```python
from build123d import *

# Parameters (mm, degrees)
F1_DEPTH = 50
F3_D     = 10
F4_SIZE  = 5
F5_SIZE  = 5.08


with BuildPart() as f1:
    # F0 (on Front) → F1 (new body)
    with BuildSketch(Plane.XZ):
        Polygon((50, 68.819096), (-50, 68.819096), (-80.901699, -26.286556), (0, -85.065081), (80.901699, -26.286556), align=None)
    extrude(amount=F1_DEPTH)

    # F3 (through all)
    with Locations(Plane(origin=(0, 0, 0), x_dir=(-1, 0, 0), z_dir=(0, 1, 0))):
        with Locations((0, 0)):
            Hole(F3_D / 2)

    # F4
    f4_edges = [f1.edges().sort_by_distance(p)[0] for p in [
        (-50, -25, 68.819096),
    ]]
    chamfer(f4_edges, length=F4_SIZE)

    # F5
    f5_edges = [f1.edges().sort_by_distance(p)[0] for p in [
        (50, -25, 68.819096),
    ]]
    chamfer(f5_edges, length=F5_SIZE)


solid = f1.part
```
Can you work these out from the model? Positions are in its coordinate system, mm. Give positions to 0.01 mm unless a question says otherwise; leave off trailing zeros. Order: outer loops, then holes, each group sorted by start corner. A loop starts at its lowest first (then second) coordinate and runs counter-clockwise, first axis right, second up. Notation, with made-up numbers: M 77.5,29.25 L 96.5,29.25 A30 ccw 96.5,61.25 Z; hole C 26,3 d8. An arc over 180 degrees is marked long. Write item = value, one per line. Start each with the question number.
Q1. Will these pins go through, and if not, where does the flat tip stop? pin 1 Ø2 at (y, z) = (-21, 6) entering from -X; pin 2 Ø8 at (x, z) = (-43, 24) entering from +Y; pin 3 Ø6 at (x, y) = (11, -26.5) entering from -Z; pin 4 Ø4 at (y, z) = (-18.5, -64) entering from +X.
Q2. Suppose I cut it at B-B (y = -7.5). Write out the boundary of the cut face in (x, z).
Q3. We'd pull the mould along X, two halves only. Please class faces 1 (the flat face through (66.44, -24.65, 18.22)), 2 (the cylindrical face through (-1.08, -25.35, -4.88)), 3 (the flat face through (1, -25, 68.819)): pulls with the +X half, pulls with the -X half, needs draft (parallel to the pull), parting line crosses it, or undercut.
Q4. Suppose I cut it at C-C (x = 53.5). Write out the boundary of the cut face in (y, z).
Q5. Suppose I cut it at A-A (z = 0). Write out the boundary of the cut face in (x, y), plus the area to 3 significant figures.
Q6. Suppose I cut it at D-D (z = 29.5). Write out the boundary of the cut face in (x, y).
Q7. I need wall thicknesses on probe 1 along Z at (x, y) = (0, -10); probe 2 along Z at (x, y) = (4.5, -21); probe 3 along Z at (x, y) = (-24.5, -31.5). Which ranges of each line are inside material? Lowest first, please. Write a range as [from, to].
Check result:
q1.pin_1 = -70.74
q1.pin_2 = 0
q1.pin_3 = -79.25
q1.pin_4 = 31.75
q2.outline = M -80.9,-26.29 L 0,-85.07 L 80.9,-26.29 L 51.57,63.99 L 44.92,68.82 L -45,68.82 L -51.55,64.06 Z; hole C 0,0 d10
q3.face_1 = pulls with the +X half
q3.face_2 = undercut
q3.face_3 = needs draft
q4.outline = M -50,-46.2 L 0,-46.2 L 0,58.05 L -50,58.05 Z
q5.outline = M -72.36,-50 L -5,-50 L -5,0 L -72.36,0 Z; M 5,-50 L 72.36,-50 L 72.36,0 L 5,0 Z
q5.area = 6,740 mm2
q6.outline = M -62.78,-50 L 62.78,-50 L 62.78,0 L -62.78,0 Z
q7.probe_1 = [-85.07, -5], [5, 68.82]
q7.probe_2 = [-81.8, -2.18], [2.18, 68.82]
q7.probe_3 = [-67.26, 68.82]
